```python
from build123d import *

# Parameters (mm, degrees)
SKETCH1_W           = 163.957
SKETCH1_H           = 163.957
SKETCH1_R           = 3.175
SKETCH1_R_2         = 76.2
BOSS_EXTRUDE1_DEPTH = 8.73125
SKETCH1_5_R         = 3.175
BOSS_EXTRUDE4_DEPTH = 9.398


with BuildPart() as part:
    # Sketch1 → Boss-Extrude1 (new body)
    with BuildSketch(Plane.XY):
        Rectangle(SKETCH1_W, SKETCH1_H)
        with Locations((-69.2785, -69.2785)):
            Circle(SKETCH1_R, mode=Mode.SUBTRACT)
        with Locations((69.2785, -69.2785)):
            Circle(SKETCH1_R, mode=Mode.SUBTRACT)
        with Locations((69.2785, 69.2785)):
            Circle(SKETCH1_R, mode=Mode.SUBTRACT)
        with Locations((-69.2785, 69.2785)):
            Circle(SKETCH1_R, mode=Mode.SUBTRACT)
        Circle(SKETCH1_R_2, mode=Mode.SUBTRACT)
        with Locations((69.2785, 69.2785)):
            Circle(SKETCH1_R)
        with Locations((-69.2785, 69.2785)):
            Circle(SKETCH1_R)
        with Locations((-69.2785, -69.2785)):
            Circle(SKETCH1_R)
        with Locations((69.2785, -69.2785)):
            Circle(SKETCH1_R)
        Circle(SKETCH1_R_2)
        with Locations((56.281763085, 9.923993354)):
            Circle(SKETCH1_R, mode=Mode.SUBTRACT)
        with Locations((-36.735311894, 43.779439924)):
            Circle(SKETCH1_R, mode=Mode.SUBTRACT)
        Circle(SKETCH1_R, mode=Mode.SUBTRACT)
        with Locations((-19.546451191, -53.703433278)):
            Circle(SKETCH1_R, mode=Mode.SUBTRACT)
        with Locations((56.281763085, 9.923993354)):
            Circle(SKETCH1_R)
        with Locations((-36.735311894, 43.779439924)):
            Circle(SKETCH1_R)
        with Locations((-19.546451191, -53.703433278)):
            Circle(SKETCH1_R)
    extrude(amount=BOSS_EXTRUDE1_DEPTH)

    # Sketch1_5 → Boss-Extrude4 (add)
    with BuildSketch(Plane.XY):
        with Locations((69.2785, 69.2785)):
            Circle(SKETCH1_5_R)
        with Locations((-69.2785, 69.2785)):
            Circle(SKETCH1_5_R)
        with Locations((-69.2785, -69.2785)):
            Circle(SKETCH1_5_R)
        with Locations((69.2785, -69.2785)):
            Circle(SKETCH1_5_R)
    extrude(amount=-BOSS_EXTRUDE4_DEPTH)


solid = part.part
```
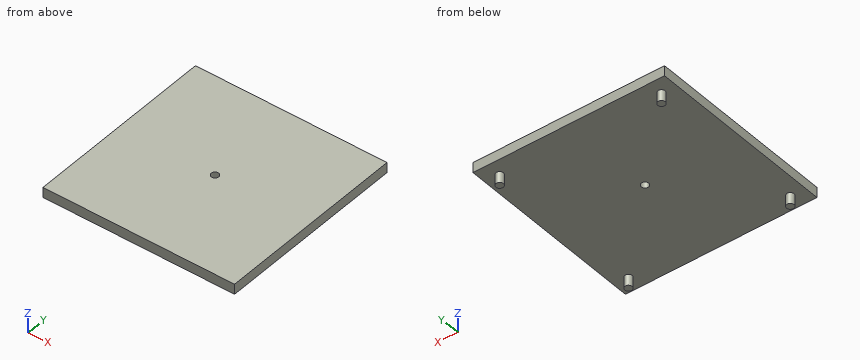
For this review, take the finished solid that the model builds, in its own axes (mm). Round coordinates to 2 decimals unless told otherwise and drop trailing zeros. Order: outer loops, then holes, each group sorted by start corner. A loop starts at its lowest first (then second) coordinate and runs counter-clockwise, first axis right, second up.
Q1. Wall thickness on line 1 (Y direction, x = 0, z = 5.5) (1 decimal); line 2 (Z direction, x = 25.5, y = -4.5); line 3 (X direction, y = -2, z = 4.5): over which ranges is each line inside the solid? List them lowest first.
Findings below:
line 1: y = -82 to -3.2, 3.2 to 82
line 2: z = 0 to 8.73
line 3: x = -81.98 to -2.47, 2.47 to 81.98
Q2. Insertion check: P1, Ø2, axis at x = -46.5, y = -16, coming from the -Z side. The pin has a flat end and moves straight along its axis. Give the tip position at first contact, or say it passes through.
Findings below:
P1: stops at z = 0
Q3. We need section A-A, the plane y = 0. Give the boundary of the cut face in (x, z) (1 decimal), plus the area to 3 significant figures.
Findings below:
outline: (-82, 0) - (-3.2, 0) - (-3.2, 8.7) - (-82, 8.7) - close; (3.2, 0) - (82, 0) - (82, 8.7) - (3.2, 8.7) - close
area: 1,380 mm2
Q4. We need section C-C, the plane y = 16.5. Give the boundary of the cut face in (x, z).
Findings below:
outline: (-81.98, 0) - (81.98, 0) - (81.98, 8.73) - (-81.98, 8.73) - close
